Autodesk Inventor part; units mm, degrees
ref_plane "YZ Plane" through (0, 0, 0) normal (1, 0, 0) x (0, 1, 0)
ref_plane "XZ Plane" through (0, 0, 0) normal (0, 1, 0) x (-1, 0, 0)
ref_plane "XY Plane" through (0, 0, 0) normal (0, 0, 1) x (1, 0, 0)
sketch "Sketch1" plane through (0, 0, 0) normal (0, 1, 0) x (-1, 0, 0)
  line L0 (49.53, 34.925) -> (-49.53, 34.925)
  line L1 (-49.53, 34.925) -> (-49.53, -34.925)
  line L2 (-49.53, -34.925) -> (49.53, -34.925)
  line L3 (49.53, -34.925) -> (49.53, 34.925)
  point P0 (0, 0)
  point P1 (0, -34.925)
  point P2 (49.53, 0)
  dimension "d0" = 99.06
  dimension "d1" = 69.85
extrude "Extrusion1" add sketch "Sketch1" along normal blind 1.778
sketch "Sketch2" plane through (0, 1.778, 0) normal (0, 1, 0) x (1, 0, 0)
  line L0 (-49.53, 34.925) -> (-49.53, -34.925)
  line L1 (-49.53, 34.925) -> (1.27, 34.925)
  line L2 (1.27, 34.925) -> (1.27, 8.763)
  line L3 (1.27, 8.763) -> (-49.53, 8.763)
  line L4 (-49.53, 8.763) -> (-49.53, 34.925)
  point P0 (0, 0)
  dimension "d4" = 50.8
  dimension "d5" = 26.162
extrude "Extrusion2" add sketch "Sketch2" along normal blind 26.162
sketch "Sketch3" plane through (0, 1.778, 0) normal (0, 1, 0) x (1, 0, 0)
  line L0 (-49.53, 34.925) -> (-49.53, -34.925)
  line L1 (-49.53, -34.925) -> (-11.43, -34.925)
  line L2 (-11.43, -34.925) -> (-11.43, -1.905)
  line L3 (-11.43, -1.905) -> (-49.53, -1.905)
  line L4 (-49.53, -1.905) -> (-49.53, -34.925)
  point P0 (0, 0)
  dimension "d8" = 38.1
  dimension "d9" = 33.02
extrude "Extrusion3" add sketch "Sketch3" along normal blind 19.05
sketch "Sketch4" plane through (0, 1.778, 0) normal (0, 1, 0) x (1, 0, 0)
  line L0 (1.27, 34.925) -> (1.27, 8.763)
  line L1 (1.27, 34.925) -> (8.89, 34.925)
  line L2 (49.53, 34.925) -> (-49.53, 34.925)
  line L3 (8.89, 34.925) -> (34.29, 34.925)
  line L4 (34.29, 34.925) -> (34.29, -15.875)
  line L5 (34.29, -15.875) -> (8.89, -15.875)
  line L6 (8.89, -15.875) -> (8.89, 34.925)
  point P0 (0, 0)
  dimension "d12" = 7.62
  dimension "d13" = 25.4
  dimension "d14" = 50.8
extrude "Extrusion4" add sketch "Sketch4" along normal blind 15.24
sketch "Sketch5" plane through (0, 0, 0) normal (0, -1, 0) x (1, 0, 0)
  line L0 (-11.43, 34.925) -> (49.53, 34.925)
  line L1 (49.53, 34.925) -> (43.18, 34.925)
  line L2 (43.18, 34.925) -> (27.94, 34.925)
  line L3 (27.94, 34.925) -> (27.94, -28.575)
  line L4 (27.94, -28.575) -> (43.18, -28.575)
  line L5 (43.18, -28.575) -> (43.18, 34.925)
  point P0 (0, 0)
  dimension "d17" = 6.35
  dimension "d18" = 15.24
  dimension "d19" = 63.5
extrude "Extrusion5" add sketch "Sketch5" along normal blind 15.24
sketch "Sketch6" plane through (0, 1.778, 0) normal (0, 1, 0) x (1, 0, 0)
  line L0 (49.53, -34.925) -> (45.7244, -34.925)
  line L1 (45.7244, -34.925) -> (57.1544, -34.925)
  line L2 (57.1544, -34.925) -> (57.1544, 23.495)
  line L3 (57.1544, 23.495) -> (45.7244, 23.495)
  line L4 (45.7244, 23.495) -> (45.7244, -34.925)
  point P0 (0, 0)
  dimension "d22" = 11.43
  dimension "d23" = 58.42
extrude "Extrusion6" add sketch "Sketch6" along normal blind 5.08
sketch "Sketch7" plane through (0, 1.778, 0) normal (0, 1, 0) x (1, 0, 0)
  line L0 (49.53, -34.925) -> (49.53, 34.925)
  line L1 (49.53, -31.9382) -> (-49.3242, -31.9382)
  line L2 (-49.3242, -31.9382) -> (-49.3242, -42.0982)
  line L3 (-49.3242, -42.0982) -> (49.53, -42.0982)
  line L4 (49.53, -42.0982) -> (49.53, -31.9382)
  point P0 (0, 0)
  dimension "d26" = 10.16
extrude "Extrusion7" add sketch "Sketch7" along normal blind 5.08
properties part number "board"
Read the model definition and answer for the solid it produces. Units are mm, in the model's axes. A direction names the side the tool comes from. Give positions to 0.01 mm unless a question says otherwise; leave off trailing zeros. Write each loop counter-clockwise with the first axis right and the second up, starting at its lowest first coordinate (ties: lowest second). Pieces come first, ordered by that corner, then holes. Notation, with made-up numbers: M 19.25,76.25 L 72.25,76.25 A30 cw 72.25,113.25 Z; hole C -22,63.25 d11. An arc over 180 degrees is marked long. Put each result on its own line as item: value. Start each with the question number.
1. The part is cut by section C-C, the plane x = 37. Give the vertices of the cut face in (y, z) (3 decimals).
2. The part is cut by section A-A, the plane y = 10.5. Give the vertices of the cut face in (x, z) (3 decimals), and give its area (3 significant figures).
3. Each of these flat-tipped pins is pushed along its axis until it touches: pin 1 Ø5.5 at (y, z) = (4, 37) entering from +X; pin 2 Ø20.5 at (x, z) = (25.5, -21.5) entering from +Y; pin 3 Ø1.5 at (x, z) = (22.5, 3.5) entering from -Y; pin 4 Ø5 at (x, y) = (30.5, -3.5) entering from -Z (3 decimals). Where does it stop, or does it pass through?
4. Which of the six approach directions +Z, -Z, +X, -X, +Y, -Y give full straight-line access (tool end or side, diameter ignored) to faces 1 (the flat face through (-31, 20.828, 18)), 2 (the flat face through (27.94, -8, 4)), 3 (the flat face through (8.89, 9, -9)), 4 (the flat face through (18, 4, 31.938))?
5. The part is cut by section D-D, the plane y = -4. Give the vertices of the cut face in (x, z) (3 decimals).
6. For a pull along X with two mould halves and no side action, classify faces 5 (the flat face through (35, -8, -28.575)), 6 (the flat face through (34.29, 9, -10)), 7 (the flat face through (45.724, 4, 4)), 8 (the flat face through (-49.53, 11, 7)) as released by +X, released by -X, zero draft, split by the parting line, or undercut.
7. Consider line 1 along X through (y, z) = (2, 11); line 2 along X through (y, z) = (8.5, -30.5); line 3 along Z through (x, y) = (-29, 13) (3 decimals). Determine where each line is inside the solid, lowest interval first.
8. The part is cut by section B-B, the plane z = 10. Give the vertices of the cut face in (x, y).
Final values:
1. outline: M -15.24,-28.575 L 0,-28.575 L 0,-34.925 L 1.778,-34.925 L 1.778,31.938 L 6.858,31.938 L 6.858,42.098 L 1.778,42.098 L 1.778,34.925 L -15.24,34.925 Z
2. outline: M -49.53,-34.925 L 1.27,-34.925 L 1.27,-8.763 L -49.53,-8.763 Z; M -49.53,1.905 L -11.43,1.905 L -11.43,34.925 L -49.53,34.925 Z; M 8.89,-34.925 L 34.29,-34.925 L 34.29,15.875 L 8.89,15.875 Z
2. area: 3,880 mm²
3. pin 1: stops at x = 57.15
3. pin 2: stops at y = 17.02
3. pin 3: stops at y = 0
3. pin 4: stops at z = -28.575
4. face 1: +Z, +X, -X, +Y
4. face 2: +Z, -Z, -X, -Y
4. face 3: -Z, +Y
4. face 4: +Y
5. outline: M 27.94,-28.575 L 43.18,-28.575 L 43.18,34.925 L 27.94,34.925 Z
6. face 5: zero draft
6. face 6: undercut
6. face 7: undercut
6. face 8: released by -X
7. line 1: x = -49.53 to -11.43, 8.89 to 34.29, 45.72 to 57.15
7. line 2: x = -49.53 to 1.27, 8.89 to 34.29
7. line 3: z = -34.925 to -8.763, 1.905 to 34.925
8. outline: M -49.53,0 L 27.94,0 L 27.94,-15.24 L 43.18,-15.24 L 43.18,0 L 49.53,0 L 49.53,1.78 L 57.15,1.78 L 57.15,6.86 L 45.72,6.86 L 45.72,1.78 L 34.29,1.78 L 34.29,17.02 L 8.89,17.02 L 8.89,1.78 L -11.43,1.78 L -11.43,20.83 L -49.53,20.83 Z
